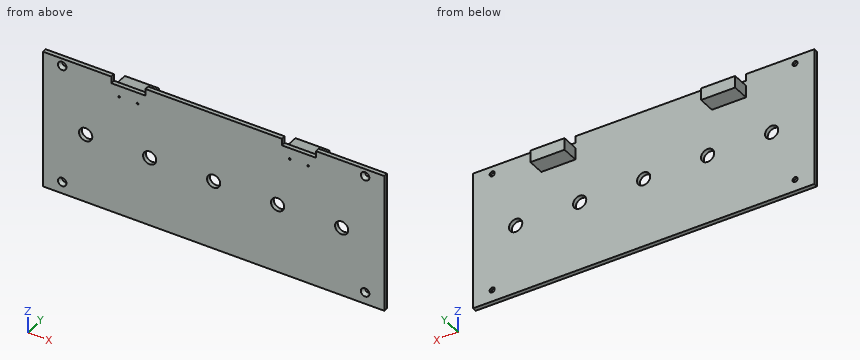
```python
from build123d import *

# Parameters (mm, degrees)
F0_W           = 203.2
F0_H           = 82.55
F1_DEPTH       = 2.54
F3_D           = 7.874
F4_DEPTH       = 25.4
F2_W           = 20.32
F2_H           = 7.112
F5_DEPTH       = 12.7
F6_D           = 3.048
F6_CSINK_D     = 5.08
F6_CSINK_ANGLE = 49
F7_D           = 1.016
F7_DEPTH       = 10.16
F7_TIP         = 0.3052371945


with BuildPart() as f1:
    # F0 (on Front) → F1 (new body)
    with BuildSketch(Plane.XZ):
        Rectangle(F0_W, F0_H)
    extrude(amount=F1_DEPTH)

    # F3 (through all)
    with Locations(Plane.XZ.offset(2.54)):
        with Locations((-76.2, 0), (-38.1, 0), (0, 0), (38.1, 0), (76.2, 0)):
            Hole(F3_D / 2)

    # F2 (on face) → F4 (cut)
    with BuildSketch(Plane.XZ.offset(2.54)):
        Polygon((-50.8, 41.275), (-40.64, 41.275), (-40.64, 45.339), (-60.96, 45.339), (-60.96, 41.275), align=None)
        Polygon((40.64, 45.339), (40.64, 41.275), (50.8, 41.275), (60.96, 41.275), (60.96, 45.339), align=None)
        Polygon((-40.64, 37.211), (-40.64, 41.275), (-50.8, 41.275), (-60.96, 41.275), (-60.96, 37.211), align=None)
        Polygon((50.8, 41.275), (40.64, 41.275), (40.64, 37.211), (60.96, 37.211), (60.96, 41.275), align=None)
    extrude(amount=-F4_DEPTH, mode=Mode.SUBTRACT)

    # F2 (on face) → F5 (join)
    with BuildSketch(Plane.XZ.offset(2.54)):
        with Locations((-50.8, 30.607)):
            Rectangle(F2_W, F2_H)
        with Locations((50.8, 30.607)):
            Rectangle(F2_W, F2_H)
    extrude(amount=-F5_DEPTH)

    # F6 (through all)
    with Locations(Plane.XZ.offset(2.54)):
        with Locations((-90.17, 36.83), (-90.17, -34.29), (90.17, 36.83), (90.17, -34.29)):
            CounterSinkHole(F6_D / 2, F6_CSINK_D / 2, counter_sink_angle=F6_CSINK_ANGLE)

    # F7
    with Locations(Plane.XZ.offset(2.54)):
        with Locations((-56.3118, 30.607), (-45.2882, 30.607), (45.2882, 30.607), (56.3118, 30.607)):
            Hole(F7_D / 2, depth=F7_DEPTH)
            with Locations((0, 0, -(F7_DEPTH + F7_TIP / 2))):  # 118° drill point
                Cone(0, F7_D / 2, F7_TIP, mode=Mode.SUBTRACT)


solid = f1.part
```
Could you check a few things on this model? Use its own coordinates, in mm. Coordinates: 2 decimals unless noted, no trailing zeros. Write each loop counter-clockwise with the first axis right and the second up, starting at its lowest first coordinate (ties: lowest second). Pieces come first, ordered by that corner, then holes. Notation, with made-up numbers: (40.5, 30.25) - (65.5, 30.25) arc R9 cw to (65.5, 41.25) - close; hole circle Ø6 at (8.5, 80). An arc over 180 degrees is marked (long way). Use a Markdown table: item, result.
Q1. Please list where these lines run through material, in increasing order: L1, parallel to X at y = -0.15, z = 36.83; L2, parallel to Z at x = 90.17, y = -0.1 (3 decimals); L3, parallel to Z at x = -38.1, y = -0.65 (3 decimals).
Geometry check:
| item | result |
|---|---|
| L1 | x = -101.6 to -91.69, -88.65 to 88.65, 91.69 to 101.6 |
| L2 | z = -41.275 to -35.814, -32.766 to 35.306, 38.354 to 41.275 |
| L3 | z = -41.275 to -3.937, 3.937 to 41.275 |
Q2. Imagine slicing it at B-B (y = 4.75). List the corners of the cut face in (x, z) for me.
Geometry check:
| item | result |
|---|---|
| outline | (-60.96, 27.05) - (-40.64, 27.05) - (-40.64, 34.16) - (-60.96, 34.16) - close; (40.64, 27.05) - (60.96, 27.05) - (60.96, 34.16) - (40.64, 34.16) - close; hole circle Ø1.02 at (-56.31, 30.61); hole circle Ø1.02 at (-45.29, 30.61); hole circle Ø1.02 at (45.29, 30.61); hole circle Ø1.02 at (56.31, 30.61) |
Q3. Imagine slicing it at A-A (x = 38.1). List the corners of the cut face in (y, z) for me (3 decimals).
Geometry check:
| item | result |
|---|---|
| outline | (-2.54, -41.275) - (0, -41.275) - (0, -3.937) - (-2.54, -3.937) - close; (-2.54, 3.937) - (0, 3.937) - (0, 41.275) - (-2.54, 41.275) - close |
Q4. I'm going to push flat-ended pins straight in: pin 1 Ø10 at (x, z) = (38.1, 0) entering from +Y; pin 2 Ø3 at (x, y) = (52.5, 6) entering from +Z; pin 3 Ø4.5 at (x, z) = (76.2, 0) entering from -Y; pin 4 Ø5.5 at (y, z) = (6.5, 32) entering from +X. Where does each tip first touch, or does it pass through?
Geometry check:
| item | result |
|---|---|
| pin 1 | stops at y = 0 |
| pin 2 | stops at z = 34.16 |
| pin 3 | passes through |
| pin 4 | stops at x = 60.96 |
Q5. Imagine slicing it at C-C (z = -17). List the corners of the cut face in (x, y) for me.
Geometry check:
| item | result |
|---|---|
| outline | (-101.6, -2.54) - (101.6, -2.54) - (101.6, 0) - (-101.6, 0) - close |
